Check sheet for the modelled part. Datum: model origin and axes. Units: mm. A direction names the side the tool comes from. Coordinates: 2 decimals unless noted, no trailing zeros. Order: outer loops, then holes, each group sorted by start corner. A loop starts at its lowest first (then second) coordinate and runs counter-clockwise, first axis right, second up.
1. Draft check along Z on faces 1 (the flat face through (-6.225, 3.042, 9.073)), 2 (the flat face through (-11.695, 3.042, -2.687)), 3 (the flat face through (-9.56, 3.04, -5.5)), 4 (the flat face through (9.37, 3.04, 7.5)). Enter one of: released by +Z, released by -Z, zero draft, split by the parting line, or undercut.
2. Cross-section at A-A (x = 0). Enter the section's corners in (y, z).
3. Gauge pin test, flat ends, axial feed: pin 1 Ø6 at (x, y) = (-3.5, 12.5) entering from +Z; pin 2 Ø5 at (x, y) = (4.5, 13) entering from +Z; pin 3 Ø3 at (y, z) = (13, -4.5) entering from -X. Record the tip position at first contact, or that the pin passes through.
4. Thickness scan on line 1 (X direction, y = 3.95, z = 0); line 2 (X direction, y = 13.75, z = 0); line 3 (Y direction, x = 8.5, z = -4.25). Record the ranges inside material, lowest first.
5. Cross-section at C-C (z = 0.5). Enter the section's corners in (x, y).
6. Cross-section at B-B (y = 13.75). Enter the section's corners in (x, z).
7. Cross-section at D-D (x = 4.5). Enter the section's corners in (y, z).
8. Set-up check for faces 5 (the flat face through (6.225, 3.042, -9.073)), 6 (the flat face through (7.5, 3, -8.1)), 7 (the flat face through (10.23, 3.04, 4.05)), 8 (the flat face through (-5.5, 6, -2.8)): record each of +Z, -Z, +X, -X, +Y, -Y from which the full face is reachable in a straight line by a thin tool's end or side.
```python
from build123d import *

# Parameters (mm, degrees)
SKETCH1_R           = 10
SKETCH1_R_2         = 3.15
BOSS_EXTRUDE1_DEPTH = 6
SKETCH2_R           = 6
SKETCH2_R_2         = 3
BOSS_EXTRUDE2_DEPTH = 10
BOSS_EXTRUDE3_DEPTH = 6


with BuildPart() as part:
    # Sketch1 → Boss-Extrude1 (new body)
    with BuildSketch(Plane(origin=(0, 0, 0), x_dir=(1, 0, 0), z_dir=(0, 1, 0))):
        Circle(SKETCH1_R)
        Circle(SKETCH1_R_2, mode=Mode.SUBTRACT)
    extrude(amount=BOSS_EXTRUDE1_DEPTH)

    # Sketch2 → Boss-Extrude2 (add)
    with BuildSketch(Plane(origin=(0, 6, 0), x_dir=(1, 0, 0), z_dir=(0, 1, 0))):
        Circle(SKETCH2_R)
        Circle(SKETCH2_R_2, mode=Mode.SUBTRACT)
    extrude(amount=BOSS_EXTRUDE2_DEPTH)

    # Sketch3 → Boss-Extrude3 (add)
    with BuildSketch(Plane(origin=(0, 6, 0), x_dir=(1, 0, 0), z_dir=(0, 1, 0))):
        with BuildLine():
            Line((1.25, 12), (-1.25, 12))
            Line((-1.25, 12), (-2.082191781, 9.780821918))
            ThreePointArc((-2.082191781, 9.780821918), (0, 10), (2.082191781, 9.780821918))
            Line((2.082191781, 9.780821918), (1.25, 12))
        make_face()
        with BuildLine():
            ThreePointArc((-6.119729557, 7.908786895), (-4.338837391, 9.009688679), (-2.367749614, 9.715645206))
            Line((-2.367749614, 9.715645206), (-4.080393785, 11.353981089))
            Line((-4.080393785, 11.353981089), (-6.332815954, 10.269271741))
            Line((-6.332815954, 10.269271741), (-6.119729557, 7.908786895))
        make_face()
        with BuildLine():
            Line((4.080393785, 11.353981089), (2.367749614, 9.715645206))
            ThreePointArc((2.367749614, 9.715645206), (4.338837391, 9.009688679), (6.119729557, 7.908786895))
            Line((6.119729557, 7.908786895), (6.332815954, 10.269271741))
            Line((6.332815954, 10.269271741), (4.080393785, 11.353981089))
        make_face()
        with BuildLine():
            ThreePointArc((-8.945179841, 4.470319633), (-7.818314825, 6.234898019), (-6.348729159, 7.726165806))
            Line((-6.348729159, 7.726165806), (-8.602615537, 8.459166975))
            Line((-8.602615537, 8.459166975), (-10.161340042, 6.504588269))
            Line((-10.161340042, 6.504588269), (-8.945179841, 4.470319633))
        make_face()
        with BuildLine():
            Line((8.602615537, 8.459166975), (6.348729159, 7.726165806))
            ThreePointArc((6.348729159, 7.726165806), (7.818314825, 6.234898019), (8.945179841, 4.470319633))
            Line((8.945179841, 4.470319633), (10.161340042, 6.504588269))
            Line((10.161340042, 6.504588269), (8.602615537, 8.459166975))
        make_face()
        with BuildLine():
            ThreePointArc((-9.998927551, 0.146450742), (-9.749279122, 2.22520934), (-9.072265032, 4.206424514))
            Line((-9.072265032, 4.206424514), (-11.420983779, 3.888911098))
            Line((-11.420983779, 3.888911098), (-11.977286114, 1.451591317))
            Line((-11.977286114, 1.451591317), (-9.998927551, 0.146450742))
        make_face()
        with BuildLine():
            Line((11.420983779, 3.888911098), (9.072265032, 4.206424514))
            ThreePointArc((9.072265032, 4.206424514), (9.749279122, 2.22520934), (9.998927551, 0.146450742))
            Line((9.998927551, 0.146450742), (11.977286114, 1.451591317))
            Line((11.977286114, 1.451591317), (11.420983779, 3.888911098))
        make_face()
        with BuildLine():
            ThreePointArc((-9.072265032, -4.206424514), (-9.749279122, -2.22520934), (-9.998927551, -0.146450742))
            Line((-9.998927551, -0.146450742), (-11.977286114, -1.451591317))
            Line((-11.977286114, -1.451591317), (-11.420983779, -3.888911098))
            Line((-11.420983779, -3.888911098), (-9.072265032, -4.206424514))
        make_face()
        with BuildLine():
            Line((11.977286114, -1.451591317), (9.998927551, -0.146450742))
            ThreePointArc((9.998927551, -0.146450742), (9.749279122, -2.22520934), (9.072265032, -4.206424514))
            Line((9.072265032, -4.206424514), (11.420983779, -3.888911098))
            Line((11.420983779, -3.888911098), (11.977286114, -1.451591317))
        make_face()
        with BuildLine():
            ThreePointArc((-6.348729159, -7.726165806), (-7.818314825, -6.234898019), (-8.945179841, -4.470319633))
            Line((-8.945179841, -4.470319633), (-10.161340042, -6.504588269))
            Line((-10.161340042, -6.504588269), (-8.602615537, -8.459166975))
            Line((-8.602615537, -8.459166975), (-6.348729159, -7.726165806))
        make_face()
        with BuildLine():
            Line((10.161340042, -6.504588269), (8.945179841, -4.470319633))
            ThreePointArc((8.945179841, -4.470319633), (7.818314825, -6.234898019), (6.348729159, -7.726165806))
            Line((6.348729159, -7.726165806), (8.602615537, -8.459166975))
            Line((8.602615537, -8.459166975), (10.161340042, -6.504588269))
        make_face()
        with BuildLine():
            ThreePointArc((-2.367749614, -9.715645206), (-4.338837391, -9.009688679), (-6.119729557, -7.908786895))
            Line((-6.119729557, -7.908786895), (-6.332815954, -10.269271741))
            Line((-6.332815954, -10.269271741), (-4.080393785, -11.353981089))
            Line((-4.080393785, -11.353981089), (-2.367749614, -9.715645206))
        make_face()
        with BuildLine():
            Line((6.332815954, -10.269271741), (6.119729557, -7.908786895))
            ThreePointArc((6.119729557, -7.908786895), (4.338837391, -9.009688679), (2.367749614, -9.715645206))
            Line((2.367749614, -9.715645206), (4.080393785, -11.353981089))
            Line((4.080393785, -11.353981089), (6.332815954, -10.269271741))
        make_face()
        with BuildLine():
            ThreePointArc((2.082191781, -9.780821918), (0, -10), (-2.082191781, -9.780821918))
            Line((-2.082191781, -9.780821918), (-1.25, -12))
            Line((-1.25, -12), (1.25, -12))
            Line((1.25, -12), (2.082191781, -9.780821918))
        make_face()
    extrude(amount=-BOSS_EXTRUDE3_DEPTH)


solid = part.part
```
Data:
1. face 1: undercut
1. face 2: released by -Z
1. face 3: undercut
1. face 4: released by +Z
2. outline: (0, -12) - (6, -12) - (6, -6) - (16, -6) - (16, -3) - (6, -3) - (6, -3.15) - (0, -3.15) - close; (0, 3.15) - (6, 3.15) - (6, 3) - (16, 3) - (16, 6) - (6, 6) - (6, 12) - (0, 12) - close
3. pin 1: stops at z = 5.98
3. pin 2: stops at z = 5.66
3. pin 3: stops at x = -5.2
4. line 1: x = -10 to -3.15, 3.15 to 10
4. line 2: x = -6 to -3, 3 to 6
4. line 3: y = 0 to 6
5. outline: (-10.53, 0) - (-3.11, 0) - (-3.11, 6) - (-2.96, 6) - (-2.96, 16) - (-5.98, 16) - (-5.98, 6) - (-10.53, 6) - close; (2.96, 6) - (3.11, 6) - (3.11, 0) - (10.53, 0) - (10.53, 6) - (5.98, 6) - (5.98, 16) - (2.96, 16) - close
6. outline: circle Ø12 at (0, 0); hole circle Ø6 at (0, 0)
7. outline: (0, -11.15) - (6, -11.15) - (6, -3.97) - (16, -3.97) - (16, 3.97) - (6, 3.97) - (6, 11.15) - (0, 11.15) - close
8. face 5: +Y, -Y
8. face 6: -Z, +Y, -Y
8. face 7: +X, +Y, -Y
8. face 8: +Y
